CAD build for the part. Positions are in the model's coordinates, mm. A direction names the side the tool comes from. Round coordinates to 2 decimals unless told otherwise and drop trailing zeros. Loops run counter-clockwise (first coordinate to the right, second up) from the corner with the lowest first, then second, coordinate; pieces in that order, holes last.
```python
from build123d import *

# Parameters (mm, degrees)
SKETCH2_R               = 15
BOSS_EXTRUDE3_DEPTH     = 10
SKETCH4_R               = 2
CUT_EXTRUDE2_DEPTH      = 21
CUT_EXTRUDE2_DEPTH_BACK = 61
BOSS_EXTRUDE5_DEPTH     = 14
SKETCH5_R               = 15
BOSS_EXTRUDE6_DEPTH     = 116
SKETCH6_W               = 30
SKETCH6_H               = 2.5
CUT_EXTRUDE3_DEPTH      = 34.5
CUT_EXTRUDE3_DEPTH_BACK = 47.5


with BuildPart() as part:
    # Sketch2 → Boss-Extrude3 (new body)
    with BuildSketch(Plane(origin=(0, 0, 0), x_dir=(1, 0, 0), z_dir=(0, 1, 0))):
        with BuildLine():
            Line((88.382622063, 30), (88.382622063, 40))
            ThreePointArc((88.382622063, 40), (62.498263852, 30.495901364), (48.914280319, 6.5))
            Line((48.914280319, 6.5), (18.914280319, 6.5))
            ThreePointArc((18.914280319, 6.5), (11.618950039, 16.278820596), (0, 20))
            Line((0, 20), (-39.7, 20))
            Line((-39.7, 20), (-39.7, 10))
            Line((-39.7, 10), (-17.320508076, 10))
            ThreePointArc((-17.320508076, 10), (-20, 0), (-17.320508076, -10))
            Line((-17.320508076, -10), (-39.7, -10))
            Line((-39.7, -10), (-39.7, -20))
            Line((-39.7, -20), (0, -20))
            ThreePointArc((0, -20), (11.618950039, -16.278820596), (18.914280319, -6.5))
            Line((18.914280319, -6.5), (48.914280319, -6.5))
            ThreePointArc((48.914280319, -6.5), (62.498263852, -30.495901364), (88.382622063, -40))
            Line((88.382622063, -40), (88.382622063, -30))
            ThreePointArc((88.382622063, -30), (58.382622063, 0), (88.382622063, 30))
        make_face()
        Circle(SKETCH2_R, mode=Mode.SUBTRACT)
    extrude(amount=BOSS_EXTRUDE3_DEPTH)

    # Sketch4 → Cut-Extrude2 (cut, two sides)
    with BuildSketch(Plane.XY.offset(20)) as cut_extrude2_sk:
        with BuildLine():
            Line((-34.7, 10), (-39.7, 10))
            Line((-39.7, 10), (-39.7, 5))
            ThreePointArc((-39.7, 5), (-38.235533906, 8.535533906), (-34.7, 10))
        make_face()
        with BuildLine():
            ThreePointArc((-34.7, 0), (-38.235533906, 1.464466094), (-39.7, 5))
            Line((-39.7, 5), (-39.7, 0))
            Line((-39.7, 0), (-34.7, 0))
        make_face()
        with Locations((-34.7, 5)):
            Circle(SKETCH4_R)
    extrude(amount=CUT_EXTRUDE2_DEPTH, mode=Mode.SUBTRACT)
    extrude(cut_extrude2_sk.sketch, amount=-CUT_EXTRUDE2_DEPTH_BACK, mode=Mode.SUBTRACT)

    # Sketch2<6> → Boss-Extrude5 (add)
    with BuildSketch(Plane(origin=(0, 0, 0), x_dir=(1, 0, 0), z_dir=(0, 1, 0))):
        with BuildLine():
            ThreePointArc((15, 0), (10.606601718, 10.606601718), (0, 15))
            Line((0, 15), (0, -15))
            ThreePointArc((0, -15), (10.606601718, -10.606601718), (15, 0))
        make_face()
        with BuildLine():
            Line((0, -15), (0, 15))
            ThreePointArc((0, 15), (-15, 0), (0, -15))
        make_face()
    extrude(amount=BOSS_EXTRUDE5_DEPTH)

    # Sketch5 → Boss-Extrude6 (add)
    with BuildSketch(Plane.XZ):
        Circle(SKETCH5_R)
    extrude(amount=BOSS_EXTRUDE6_DEPTH)

    # Sketch6 → Cut-Extrude3 (cut, two sides)
    with BuildSketch(Plane.XY.offset(6.5)) as cut_extrude3_sk:
        with Locations((33.914280319, 8.75)):
            Rectangle(SKETCH6_W, SKETCH6_H)
        with Locations((33.914280319, 1.25)):
            Rectangle(SKETCH6_W, SKETCH6_H)
    extrude(amount=CUT_EXTRUDE3_DEPTH, mode=Mode.SUBTRACT)
    extrude(cut_extrude3_sk.sketch, amount=-CUT_EXTRUDE3_DEPTH_BACK, mode=Mode.SUBTRACT)


solid = part.part
```
Item 1: Two-plate mould, pull along X, no slides. Class faces 6 (the flat face through (58, 0, 0)), 7 (the cylindrical face through (11.477, 4.93, 16.379)), 8 (the cylindrical face through (58.39, 4.93, 0.66)): released by +X, released by -X, zero draft, split by the parting line, or undercut.
Answers follow:
face 6: zero draft
face 7: undercut
face 8: released by +X
Item 2: Cut at A-A, the plane x = -6. Give the cut face in (y, z).
Answers follow:
outline: (-116, -13.75) - (0, -13.75) - (0, -20) - (10, -20) - (10, -13.75) - (14, -13.75) - (14, 13.75) - (10, 13.75) - (10, 20) - (0, 20) - (0, 13.75) - (-116, 13.75) - close
Item 3: Flat gauge pins, fed straight in: P1, Ø3, axis at x = -11, y = 7, coming from the +Z side; P2, Ø4, axis at x = 29.5, z = 2, coming from the +Y side; P3, Ø5, axis at x = -26.5, y = 3, coming from the -Z side. Where does each tip first touch, or does it go through?
Answers follow:
P1: stops at z = 20
P2: stops at y = 7.5
P3: stops at z = -20
Item 4: Cut at D-D, the plane z = 25. Give the cut face in (x, y), plus the area to 3 significant figures.
Answers follow:
outline: (57.16, 0) - (71.8, 0) - (71.8, 10) - (57.16, 10) - close
area: 146 mm2
Item 5: Cut at B-B, the plane y = -92. Give the cut face in (x, z).
Answers follow:
outline: circle Ø30 at (0, 0)
Item 6: Cut at C-C, the plane z = -4. Give the cut face in (x, y).
Answers follow:
outline: (-19.6, 0) - (-14.46, 0) - (-14.46, -116) - (14.46, -116) - (14.46, 0) - (18.91, 0) - (18.91, 2.5) - (48.91, 2.5) - (48.91, 0) - (58.65, 0) - (58.65, 10) - (48.91, 10) - (48.91, 7.5) - (18.91, 7.5) - (18.91, 10) - (14.46, 10) - (14.46, 14) - (-14.46, 14) - (-14.46, 10) - (-19.6, 10) - close
Item 7: 3-axis set-ups, long thin cutter, end or side, ignore diameter. For faces 1 (the flat face through (-14, 0, 9)), 2 (the flat face through (-20, 5, -20)), 3 (the flat face through (34, 2.5, 0)), 4 (the flat face through (34, 5, -6.5)), 5 (the flat face through (34, 7.5, 0)): which of +Z, -Z, +X, -X, +Y, -Y reach the whole face in a straight line?
Answers follow:
face 1: -Y
face 2: -Z, -X, +Y, -Y
face 3: +Z, -Z, -Y
face 4: -Z, +Y, -Y
face 5: +Z, -Z, +Y
Item 8: Probe line 1 (Y direction, x = -34.7, z = 18); line 2 (X direction, y = -53.5, z = 0.5); line 3 (Y direction, x = 56, z = -14.5). List the from-to ranges inside material, lowest first.
Answers follow:
line 1: y = 0 to 3, 7 to 10
line 2: x = -14.99 to 14.99
line 3: y = 0 to 10
